Here's how the part is built. I have some questions about the finished solid (model axes, mm). Face numbers are marked on the shaded views. Coordinates: 2 decimals unless noted, no trailing zeros. Loops run counter-clockwise (first coordinate to the right, second up) from the corner with the lowest first, then second, coordinate; pieces in that order, holes last. Notation, with made-up numbers: (-23, -38.75) -> (-5, -38.75) arc R23 cw to (-5, -4.75) -> close; hole circle Ø4 at (39, 32.25). An arc over 180 degrees is marked (long way). Answer as a JSON object with one key per item and string values. Group by question number.
1) If we mould it in two halves opening along Y, with no side actions, what happens to the marked faces 1, 2 and 3? For each: +Y half, -Y half, draft (parallel to the pull), parting line (faces both ways), or undercut.
2) I want a section at D-D (y = -10.75). Write out the boundary of the cut face in (x, z).
3) I want a section at B-B (y = 11). Write out the boundary of the cut face in (x, z), then the cut area to 3 significant figures.
4) I need wall thicknesses on probe 1 along Y at (x, z) = (3, 1.55); probe 2 along Y at (x, z) = (4.5, 1.55); probe 3 along X at (y, z) = (-1.25, 1.65). Which ranges of each line are inside material? Lowest first, please. Write a range as [from, to].
5) I want a section at C-C (x = 3). Write out the boundary of the cut face in (y, z), then the cut area to 3 significant figures.
6) I want a section at A-A (z = 0.85). Write out the boundary of the cut face in (x, y).
```python
from build123d import *

# Parameters (mm, degrees)
ESBO_O1_W                = 8
ESBO_O1_H                = 29
ESBO_O1_R                = 1.65
RESSALTO_EXTRUS_O1_DEPTH = 3


with BuildPart() as part:
    # Esboço1 → Ressalto-extrusão1 (new body)
    with BuildSketch(Plane.XY):
        with Locations((4, 0)):
            Rectangle(ESBO_O1_W, ESBO_O1_H)
        with Locations((3, 11)):
            Circle(ESBO_O1_R, mode=Mode.SUBTRACT)
        with Locations((3, 0)):
            Circle(ESBO_O1_R, mode=Mode.SUBTRACT)
        with Locations((3, -11)):
            Circle(ESBO_O1_R, mode=Mode.SUBTRACT)
    extrude(amount=RESSALTO_EXTRUS_O1_DEPTH)


solid = part.part
```
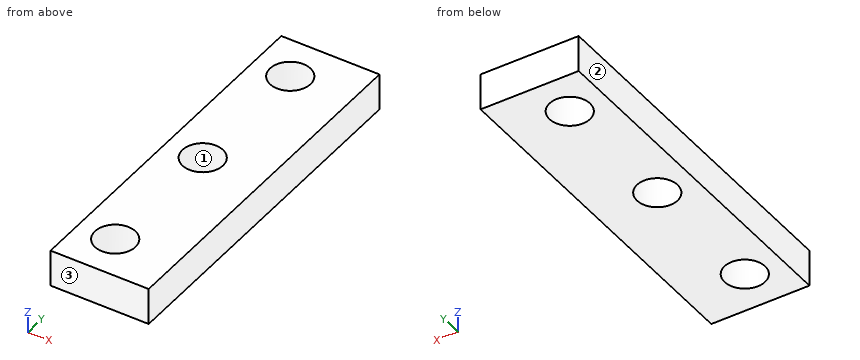
Determined:
{
 "1": {"face 1": "undercut", "face 2": "draft", "face 3": "-Y half"},
 "2": {"outline": "(0, 0) -> (1.37, 0) -> (1.37, 3) -> (0, 3) -> close; (4.63, 0) -> (8, 0) -> (8, 3) -> (4.63, 3) -> close"},
 "3": {"outline": "(0, 0) -> (1.35, 0) -> (1.35, 3) -> (0, 3) -> close; (4.65, 0) -> (8, 0) -> (8, 3) -> (4.65, 3) -> close", "area": "14.1 mm^2"},
 "4": {"probe 1": "[-14.5, -12.65], [-9.35, -1.65], [1.65, 9.35], [12.65, 14.5]", "probe 2": "[-14.5, -11.69], [-10.31, -0.69], [0.69, 10.31], [11.69, 14.5]", "probe 3": "[0, 1.92], [4.08, 8]"},
 "5": {"outline": "(-14.5, 0) -> (-12.65, 0) -> (-12.65, 3) -> (-14.5, 3) -> close; (-9.35, 0) -> (-1.65, 0) -> (-1.65, 3) -> (-9.35, 3) -> close; (1.65, 0) -> (9.35, 0) -> (9.35, 3) -> (1.65, 3) -> close; (12.65, 0) -> (14.5, 0) -> (14.5, 3) -> (12.65, 3) -> close", "area": "57.3 mm^2"},
 "6": {"outline": "(0, -14.5) -> (8, -14.5) -> (8, 14.5) -> (0, 14.5) -> close; hole circle Ø3.3 at (3, -11); hole circle Ø3.3 at (3, 0); hole circle Ø3.3 at (3, 11)"}
}
